Answer from the drawing. Dimensions are ordinates in mm from the lowest x, y and z of the part. Round coordinates to 2 decimals unless told otherwise and drop trailing zeros. Write each loop counter-clockwise with the first axis right and the second up, starting at its lowest first coordinate (ties: lowest second). Pieces come first, ordered by that corner, then holes. Notation, with made-up numbers: (89.5, -5) - (140.5, -5) arc R18 cw to (140.5, 29) - close; hole circle Ø1 at (15, 50.25). An arc over 180 degrees is marked (long way). Answer as a JSON object with one key per item and string values.
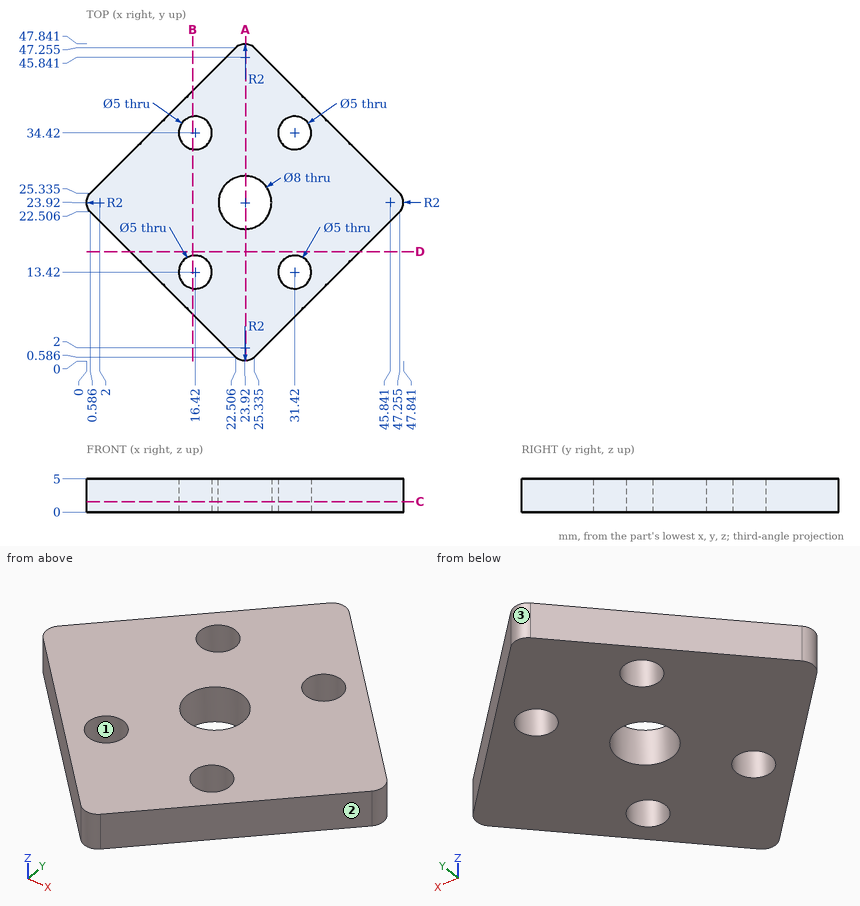
Item 1: A cutting plane is placed at B-B (x = 16). Write down the section's boundary in (y, z) (1 decimal), and give its area (3 significant figures).
Results found:
{"outline": "(7.1, 0) - (11, 0) - (11, 5) - (7.1, 5) - close; (15.9, 0) - (32, 0) - (32, 5) - (15.9, 5) - close; (36.9, 0) - (40.7, 0) - (40.7, 5) - (36.9, 5) - close", "area": "119 mm²"}
Item 2: A cutting plane is placed at C-C (z = 1.6). Write down the section's boundary in (x, y) (1 decimal), and give its area (3 significant figures).
Results found:
{"outline": "(0.6, 22.5) - (22.5, 0.6) arc R2 ccw to (25.3, 0.6) - (47.3, 22.5) arc R2 ccw to (47.3, 25.3) - (25.3, 47.3) arc R2 ccw to (22.5, 47.3) - (0.6, 25.3) arc R2 ccw to start; hole circle Ø5 at (16.4, 13.4); hole circle Ø5 at (16.4, 34.4); hole circle Ø8 at (23.9, 23.9); hole circle Ø5 at (31.4, 13.4); hole circle Ø5 at (31.4, 34.4)", "area": "1,090 mm²"}
Item 3: Consider line 1 along Y through (x, z) = (24, 3.05); line 2 along Y through (x, z) = (22, 2.2); line 3 along X through (y, z) = (22.5, 0.5). Determine where each line is inside the solid, lowest interval first.
Results found:
{"line 1": "0 to 19.92, 27.92 to 47.84", "line 2": "1.09 to 20.41, 27.43 to 46.75", "line 3": "0.59 to 20.18, 27.66 to 47.25"}
Item 4: Determine the mould class of the marked faces 1, 2 and 3 for opening direction X: pulls with the +X half, pulls with the -X half, needs draft (parallel to the pull), parting line crosses it, or undercut.
Results found:
{"face 1": "undercut", "face 2": "pulls with the +X half", "face 3": "parting line crosses it"}
Item 5: A cutting plane is placed at A-A (x = 24). Write down the section's boundary in (y, z).
Results found:
{"outline": "(0, 0) - (19.92, 0) - (19.92, 5) - (0, 5) - close; (27.92, 0) - (47.84, 0) - (47.84, 5) - (27.92, 5) - close"}
Item 6: Each of these flat-tipped pins is pushed along its axis until it touches: P1, Ø3, axis at y = 18.5, z = 3, coming from the -X side; P2, Ø3, axis at y = 10, z = 2, coming from the -X side. Where does it stop, or does it pass through?
Results found:
{"P1": "x = 3.09", "P2": "x = 11.59"}
Item 7: A cutting plane is placed at D-D (y = 16.5). Write down the section's boundary in (x, z), and give its area (3 significant figures).
Results found:
{"outline": "(6.59, 0) - (41.25, 0) - (41.25, 5) - (6.59, 5) - close", "area": "173 mm²"}
